Verification items for the finished model (mm, model axes). Face numbers are marked on the shaded views. Coordinates: 2 decimals unless noted, no trailing zeros. Order: outer loops, then holes, each group sorted by start corner. A loop starts at its lowest first (then second) coordinate and runs counter-clockwise, first axis right, second up. Notation, with made-up numbers: (-6.5, 45.25) - (31.5, 45.25) arc R23 ccw to (31.5, 56.25) - close; hole circle Ø2 at (8, 4.5). An arc over 180 degrees is marked (long way). Answer as CSV lines item,"result". Start each with the question number.
1. Mould release check, pull along Z, two halves, no side actions. Record for the marked faces 1, 2 and 3: pulls with the +Z half, pulls with the -Z half, needs draft (parallel to the pull), parting line crosses it, or undercut.
2. Section check D-D (z = 6). Record the cut outline in (x, y), and give its area (3 significant figures).
3. Go/stop test with flat-tipped pins: pin 1 (6 mm diameter, centred on x = -2.5, y = -10, fed in from +Z); pin 2 (4 mm diameter, centred on y = 0, z = 0, fed in from -X); pin 3 (5 mm diameter, centred on x = -5, z = -8, fed in from +Y); pin 4 (5 mm diameter, centred on x = 0.5, y = 10, fed in from -Z). Record where each tip stops, or that it passes through.
4. Section check A-A (y = 0). Record the cut outline in (x, z) (3 decimals), and give its area (3 significant figures).
5. Section check C-C (x = -2). Record the cut outline in (y, z) (3 decimals), and give its area (3 significant figures).
6. Material ranges on L1, parallel to X at y = -3.25, z = -11.5; L2, parallel to Y at x = 2.25, z = 0 (3 decimals); L3, parallel to Z at x = -4, y = 1, recorded low to high. Write a range as [from, to].
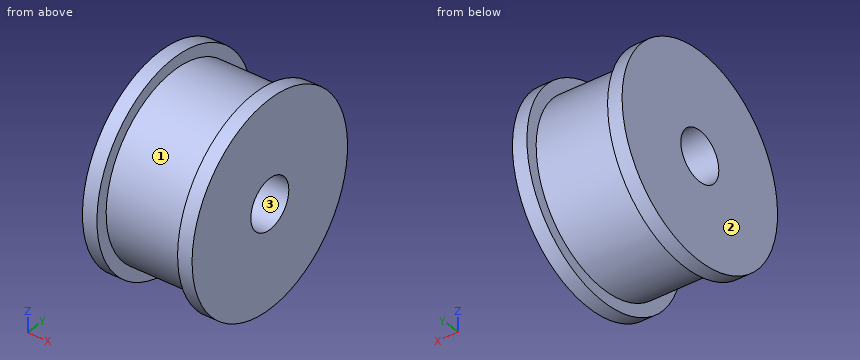
from build123d import *

# Parameters (mm, degrees)
F_1_4_0_25_DIAMETER_HOLE1_D = 6.35


with BuildPart() as part:
    # Sketch1 → Revolve1 (revolve)
    with BuildSketch(Plane(origin=(0, 0, 0), x_dir=(1, 0, 0), z_dir=(0, 1, 0))):
        Polygon((0, -11.46), (-5.15, -11.46), (-5.15, -13), (-7, -13), (-7, 0), (7, 0), (7, -13), (5.15, -13), (5.15, -11.46), align=None)
    revolve(axis=Axis((-7, 0, 0), (1, 0, 0)))

    # 1/4 (0.25) Diameter Hole1 (through all)
    with Locations(Plane.ZY.offset(7)):
        with Locations((0, 0)):
            Hole(F_1_4_0_25_DIAMETER_HOLE1_D / 2)


solid = part.part
Evaluation:
1,face 1,"parting line crosses it"
1,face 2,"needs draft"
1,face 3,"undercut"
2,outline,"(-7, -11.53) - (-5.15, -11.53) - (-5.15, -9.76) - (5.15, -9.76) - (5.15, -11.53) - (7, -11.53) - (7, 11.53) - (5.15, 11.53) - (5.15, 9.76) - (-5.15, 9.76) - (-5.15, 11.53) - (-7, 11.53) - close"
2,area,"286 mm²"
3,pin 1,"stops at z = 9.75"
3,pin 2,"passes through"
3,pin 3,"stops at y = 11.78"
3,pin 4,"stops at z = -8.66"
4,outline,"(-7, -13) - (-5.15, -13) - (-5.15, -11.46) - (5.15, -11.46) - (5.15, -13) - (7, -13) - (7, -3.175) - (-7, -3.175) - close; (-7, 3.175) - (7, 3.175) - (7, 13) - (5.15, 13) - (5.15, 11.46) - (-5.15, 11.46) - (-5.15, 13) - (-7, 13) - close"
4,area,"243 mm²"
5,outline,"circle Ø22.92 at (0, 0); hole circle Ø6.35 at (0, 0)"
5,area,"381 mm²"
6,L1,"x = [-7, -5.15], [5.15, 7]"
6,L2,"y = [-11.46, -3.175], [3.175, 11.46]"
6,L3,"z = [-11.42, -3.01], [3.01, 11.42]"
